The listing builds one solid part. Answer for the finished solid, in the listing's coordinates (mm). A direction names the side the tool comes from. Coordinates: 2 decimals unless noted, no trailing zeros. Order: outer loops, then holes, each group sorted by start corner. A loop starts at its lowest first (then second) coordinate and runs counter-clockwise, first axis right, second up. Notation, with made-up numbers: (13, 11) - (47, 11) arc R29 ccw to (47, 43) - close; hole circle Ø5 at (81, -34.5). An arc over 180 degrees is marked (long way). Use one line per item in the form item = value. Start each with the question number.
Item 1: A tool of negligible diameter and unlimited length cuts with its end or side. For faces 4 (the flat face through (-1, 2.5, 20)), 5 (the cylindrical face through (0.04, -1.27, 9.94)), 6 (the flat face through (-7, 0, 35)), 7 (the cylindrical face through (-16.65, 5.92, 4.93)), 8 (the flat face through (-11, 0, 20)), from which of +Z, -Z, +X, -X, +Y, -Y can it reach the whole face along a straight path? Write none if from no direction.
Item 2: Each of these flat-tipped pins is pushed along its axis until it touches: pin 1 Ø11 at (x, z) = (-2, 19.5) entering from +Y; pin 2 Ø5.5 at (y, z) = (0, 35.5) entering from -X; pin 3 Ø1.5 at (y, z) = (3, 27.5) entering from +X. Where does it stop, or does it pass through?
Item 3: The mould has two halves that part along Z. Classify faces 1 (the flat face through (7, -1, 20)), 2 (the conical face through (1.58, 0.121, 34.095)), 3 (the flat face through (-11, 0, 30)): released by +Z, released by -Z, zero draft, split by the parting line, or undercut.
Item 4: Consider line 1 along Z through (x, y) = (-0.5, -1.4); line 2 along X through (y, z) = (-1.4, 32.5); line 3 along Z through (x, y) = (-9.5, -0.5). Determine where each line is inside the solid, lowest interval first. Write a range as [from, to].
Item 5: Section C-C, the plane y = 2 is taken. Write down the section's boundary in (x, z).
Item 6: Section D-D, the plane z = 32.5 is taken. Write down the section's boundary in (x, y).
Item 7: Section B-B, the plane x = -0.5 is taken. Write down the section's boundary in (y, z).
Item 8: Section A-A, the plane z = 7.5 is taken. Write down the section's boundary in (x, y), and give its area (3 significant figures).
from build123d import *

# Parameters (mm, degrees)
SKETCH_1_W                = 14
SKETCH_1_H                = 5
EXTRUDE_1_DEPTH           = 40
SKETCH_3_R                = 2.5
EXTRUDE_2_DEPTH           = 40
CUT_EXTRUDE_1_DEPTH       = 10
PATTERN_LINEAR_1_COUNT    = 2
PATTERN_LINEAR_1_PITCH    = 20
HOLE_WIZARD_1_D           = 5
HOLE_WIZARD_1_CSINK_D     = 10
HOLE_WIZARD_1_CSINK_ANGLE = 90
CHAMFER_2_SIZE            = 1.5


with BuildPart() as part:
    # 草图1 → 凸台-拉伸1 (new body)
    with BuildSketch(Plane.XY):
        Rectangle(SKETCH_1_W, SKETCH_1_H)
    extrude(amount=EXTRUDE_1_DEPTH)

    # 草图3 → 凸台-拉伸2 (add)
    with BuildSketch(Plane(origin=(0, 0, 0), x_dir=(-1, 0, 0), z_dir=(0, 0, -1))):
        with BuildLine():
            Line((8, 2.5), (7, 2.5))
            Line((7, 2.5), (7, -2.5))
            Line((7, -2.5), (13, -2.5))
            ThreePointArc((13, -2.5), (16.535533906, 6.035533906), (8, 2.5))
        make_face()
        with Locations((13, 2.5)):
            Circle(SKETCH_3_R, mode=Mode.SUBTRACT)
    extrude(amount=-EXTRUDE_2_DEPTH)

    # 草图4 → 切除-拉伸1 (cut)
    with BuildSketch(Plane.XY.offset(40)):
        Polygon((-7, 2.5), (-7, 10.867672428), (-20.063850781, 10.867672428), (-20.063850781, -3.934204251), (-7, -3.934204251), align=None)
    cut_extrude_1 = extrude(amount=-CUT_EXTRUDE_1_DEPTH, mode=Mode.SUBTRACT)

    # 阵列(线性)1: 切除-拉伸1 ×2
    with Locations(*[(0, 0, -i * PATTERN_LINEAR_1_PITCH) for i in range(1, PATTERN_LINEAR_1_COUNT)]):
        add(cut_extrude_1, mode=Mode.SUBTRACT)

    # 打孔尺寸(%根据十字)槽半沉头木螺钉的类型1 (through all)
    with Locations(Plane(origin=(0, 2.5, 0), x_dir=(1, 0, 0), z_dir=(0, 1, 0))):
        with Locations((-0.5, -32.5), (-0.5, -7.5)):
            CounterSinkHole(HOLE_WIZARD_1_D / 2, HOLE_WIZARD_1_CSINK_D / 2, counter_sink_angle=HOLE_WIZARD_1_CSINK_ANGLE)

    # 倒角2
    chamfer_2_edges = [part.edges().sort_by_distance(p)[0] for p in [
        (7, 2.5, 20),
    ]]
    chamfer(chamfer_2_edges, length=CHAMFER_2_SIZE)


solid = part.part
Response:
q1.face_4 = +Z, -Z, +X, +Y
q1.face_5 = +Y, -Y
q1.face_6 = +Z, -X, +Y, -Y
q1.face_7 = +Z, -Z
q1.face_8 = -X, +Y, -Y
q2.pin_1 = 2.5
q2.pin_2 = -7
q2.pin_3 = 5.75
q3.face_1 = zero draft
q3.face_2 = undercut
q3.face_3 = released by +Z
q4.line_1 = [0, 5], [10, 30], [35, 40]
q4.line_2 = [-7, -3], [2, 7]
q4.line_3 = [0, 10], [20, 30]
q5.outline = (-17.97, 0) - (-15.45, 0) - (-15.45, 10) - (-17.97, 10) - close; (-17.97, 20) - (-15.45, 20) - (-15.45, 30) - (-17.97, 30) - close; (-10.55, 0) - (6, 0) - (6, 40) - (-7, 40) - (-7, 30) - (-10.55, 30) - (-10.55, 20) - (-7, 20) - (-7, 10) - (-10.55, 10) - close; hole circle Ø9 at (-0.5, 7.5); hole circle Ø9 at (-0.5, 32.5)
q6.outline = (-7, -2.5) - (-3, -2.5) - (-3, 0) - (-5.5, 2.5) - (-7, 2.5) - close; (2, -2.5) - (7, -2.5) - (7, 1) - (5.5, 2.5) - (4.5, 2.5) - (2, 0) - close
q7.outline = (-2.5, 0) - (2.5, 0) - (2.5, 2.5) - (0, 5) - (-2.5, 5) - close; (-2.5, 10) - (0, 10) - (2.5, 12.5) - (2.5, 27.5) - (0, 30) - (-2.5, 30) - close; (-2.5, 35) - (0, 35) - (2.5, 37.5) - (2.5, 40) - (-2.5, 40) - close
q8.outline = (-13, -2.5) - (-3, -2.5) - (-3, 0) - (-5.5, 2.5) - (-8, 2.5) arc R5 ccw (long way) to start; (2, -2.5) - (7, -2.5) - (7, 1) - (5.5, 2.5) - (4.5, 2.5) - (2, 0) - close; hole circle Ø5 at (-13, 2.5)
q8.area = 107 mm2
